Geometry check sheet. Reference: the model listing, model coordinates, mm. Face numbers are marked on the shaded views. A direction names the side the tool comes from. Give positions to 0.01 mm unless a question says otherwise; leave off trailing zeros. Order: outer loops, then holes, each group sorted by start corner. A loop starts at its lowest first (then second) coordinate and runs counter-clockwise, first axis right, second up. Notation, with made-up numbers: M -2.75,78.5 L 13.25,78.5 A6 cw 13.25,87.5 Z; hole C 49.5,-27 d2. An arc over 180 degrees is marked long. Answer as a JSON object with one key per item and string values. Group by question number.
from build123d import *

# Parameters (mm, degrees)
SKETCH1_R            = 36.5125
SKETCH1_R_2          = 30.1625
RIM_DEPTH            = 9.525
SKETCH2_R            = 30.1625
INNER_HUB_DEPTH      = 2.54
INNER_HUB_DEPTH_BACK = 2.54
SKETCH3_R            = 11.1125
HEX_STEP_DEPTH       = 1.27


with BuildPart() as part:
    # Sketch1 → Rim (new body)
    with BuildSketch(Plane(origin=(0, 0, 0), x_dir=(1, 0, 0), z_dir=(0, 1, 0))):
        Circle(SKETCH1_R)
        Circle(SKETCH1_R_2, mode=Mode.SUBTRACT)
    extrude(amount=RIM_DEPTH)

    # Sketch2 → Inner_Hub (add, two sides)
    with BuildSketch(Plane(origin=(0, 4.7625, 0), x_dir=(1, 0, 0), z_dir=(0, 1, 0))) as inner_hub_sk:
        Circle(SKETCH2_R)
        Polygon((7.200760698, 1.382887815), (2.402764371, 6.927485598), (-4.797996327, 5.544597783), (-7.200760698, -1.382887815), (-2.402764371, -6.927485598), (4.797996327, -5.544597783), align=None, mode=Mode.SUBTRACT)
    extrude(amount=INNER_HUB_DEPTH)
    extrude(inner_hub_sk.sketch, amount=-INNER_HUB_DEPTH_BACK)

    # Sketch3 → Hex_Step (add)
    with BuildSketch(Plane.XZ.offset(-2.2225)):
        Circle(SKETCH3_R)
        Polygon((4.797996327, 5.544597783), (-2.402764371, 6.927485598), (-7.200760698, 1.382887815), (-4.797996327, -5.544597783), (2.402764371, -6.927485598), (7.200760698, -1.382887815), align=None, mode=Mode.SUBTRACT)
    hex_step = extrude(amount=HEX_STEP_DEPTH)

    # Mirror1: Hex_Step across plane
    add(hex_step.mirror(Plane.ZX.offset(4.7625)))


solid = part.part
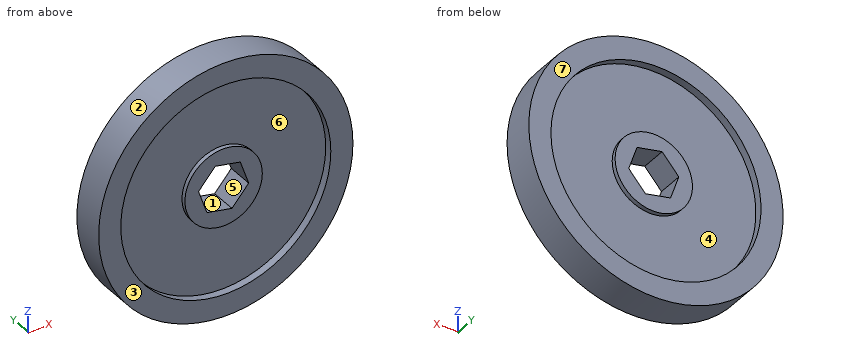
1. Cross-section at C-C (z = 0). Record the cut outline in (x, y) (1 decimal).
2. Cross-section at D-D (x = -26). Record the cut outline in (y, z) (1 decimal), and give its area (3 significant figures).
3. Cross-section at A-A (y = 6). Record the cut outline in (x, z) (1 decimal).
4. Cross-section at B-B (x = -0.5). Record the cut outline in (y, z) (1 decimal), and give its area (3 significant figures).
5. Access from +Z, -Z, +X, -X, +Y, -Y to the whole of each face (thin tool, end or side, straight path). Record for the marked faces 4, 5, 6 and 7.
6. Release check for a two-part mould opening along Z. For the marked faces 1, 2 and 3 record: released by +Z, released by -Z, zero draft, split by the parting line, or undercut.
7. Thickness scan on line 1 along X through (y, z) = (8.95, 0); line 2 along Z through (x, y) = (0, 8.15); line 3 along X through (y, z) = (1.5, -3). Record the ranges inside material, lowest first. Write a range as [from, to].
8. Depth check by flat-ended pin: pin 1 (6.5 mm diameter, centred on x = 0.5, z = 1.5, fed in from -Y); pin 2 (3 mm diameter, centred on x = 19, y = 5.5, fed in from -Z); pin 3 (5 mm diameter, centred on x = 5, y = 5, fed in from +Z); pin 4 (1 mm diameter, centred on x = 17, y = 2, fed in from -Z). Enter the tip coordinate at first touch or a pass-through.
Report:
{
 "1": {"outline": "M -36.5,0 L -30.2,0 L -30.2,2.2 L -11.1,2.2 L -11.1,1 L -6.7,1 L -6.7,8.6 L -11.1,8.6 L -11.1,7.3 L -30.2,7.3 L -30.2,9.5 L -36.5,9.5 Z; M 6.7,1 L 11.1,1 L 11.1,2.2 L 30.2,2.2 L 30.2,0 L 36.5,0 L 36.5,9.5 L 30.2,9.5 L 30.2,7.3 L 11.1,7.3 L 11.1,8.6 L 6.7,8.6 Z"},
 "2": {"outline": "M 0,-25.6 L 9.5,-25.6 L 9.5,-15.3 L 7.3,-15.3 L 7.3,15.3 L 9.5,15.3 L 9.5,25.6 L 0,25.6 L 0,15.3 L 2.2,15.3 L 2.2,-15.3 L 0,-15.3 Z", "area": "352 mm2"},
 "3": {"outline": "C 0,0 d73; hole M -7.2,1.4 L -4.8,-5.5 L 2.4,-6.9 L 7.2,-1.4 L 4.8,5.5 L -2.4,6.9 Z"},
 "4": {"outline": "M 0,-36.5 L 9.5,-36.5 L 9.5,-30.2 L 7.3,-30.2 L 7.3,-11.1 L 8.6,-11.1 L 8.6,-6.4 L 1,-6.4 L 1,-11.1 L 2.2,-11.1 L 2.2,-30.2 L 0,-30.2 Z; M 0,30.2 L 2.2,30.2 L 2.2,11.1 L 1,11.1 L 1,6.6 L 8.6,6.6 L 8.6,11.1 L 7.3,11.1 L 7.3,30.2 L 9.5,30.2 L 9.5,36.5 L 0,36.5 Z", "area": "385 mm2"},
 "5": {"face 4": "+Y", "face 5": "+Y, -Y", "face 6": "-Y", "face 7": "+Z, -Z, +X, -X, +Y"},
 "6": {"face 1": "undercut", "face 2": "split by the parting line", "face 3": "zero draft"},
 "7": {"line 1": "x = [-36.51, -30.16], [30.16, 36.51]", "line 2": "z = [-36.51, -30.16], [-11.11, -6.47], [6.47, 11.11], [30.16, 36.51]", "line 3": "x = [-36.39, -30.01], [-10.7, -5.68], [5.8, 10.7], [30.01, 36.39]"},
 "8": {"pin 1": "passes through", "pin 2": "stops at z = -32.05", "pin 3": "stops at z = 36.43", "pin 4": "stops at z = -32.57"}
}
